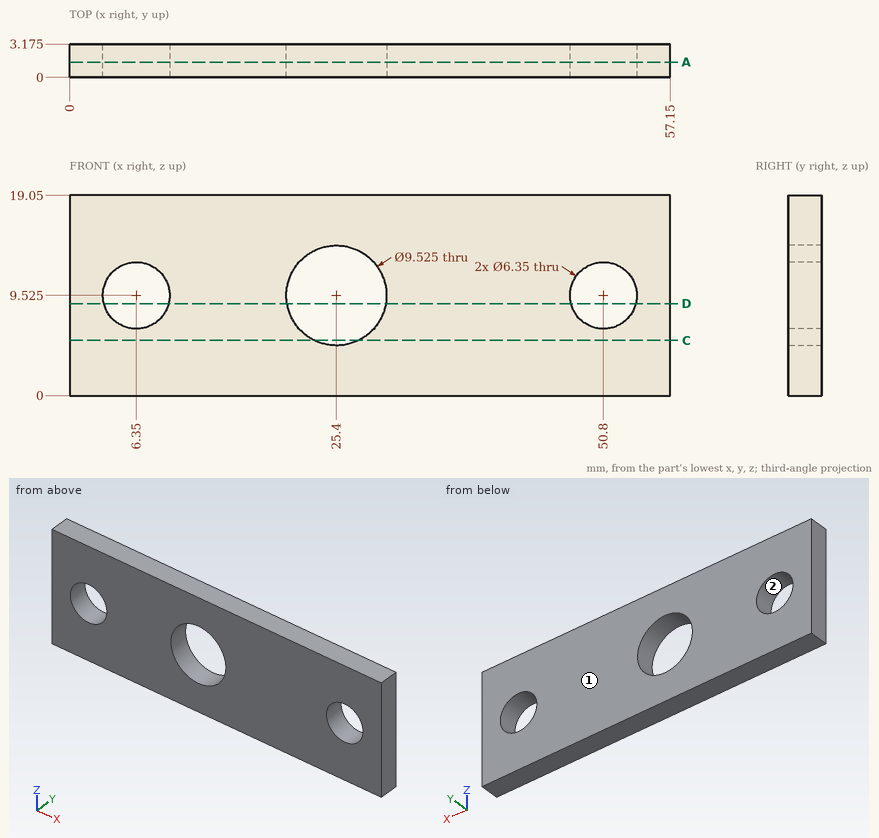
Answer from the drawing. Dimensions are ordinates in mm from the lowest x, y and z of the part. Give positions to 0.01 mm unless a question says otherwise; leave off trailing zeros. Loops run counter-clockwise (first coordinate to the right, second up) from the corner with the lowest first, then second, coordinate; pieces in that order, holes last.
Item 1: The part is cut by section A-A (y = 1.45). Give the number of separate pieces and of enclosed holes in the cut face, and give its area (3 significant figures).
Item 2: The part is cut by section C-C (z = 5.25). Write down the section's boundary in (x, y) (3 decimals).
Item 3: The part is cut by section D-D (z = 8.75). Write down the section's boundary in (x, y) (3 decimals).
Item 4: The mould has two halves that part along X. Classify the marked faces 1 and 2: released by +X, released by -X, zero draft, split by the parting line, or undercut.
Item 5: Find the intervals of material crossed by line 1 along X through (y, z) = (0.5, 9.5); line 2 along Z through (x, y) = (25.5, 0.1); line 3 along X through (y, z) = (1.8, 8.5) (3 decimals), in increasing order.
Taken from the geometry:
1. separate pieces: 1
1. enclosed holes: 3
1. area: 954 mm2
2. outline: (0, 0) - (23.301, 0) - (23.301, 3.175) - (0, 3.175) - close; (27.499, 0) - (57.15, 0) - (57.15, 3.175) - (27.499, 3.175) - close
3. outline: (0, 0) - (3.271, 0) - (3.271, 3.175) - (0, 3.175) - close; (9.429, 0) - (20.701, 0) - (20.701, 3.175) - (9.429, 3.175) - close; (30.099, 0) - (47.721, 0) - (47.721, 3.175) - (30.099, 3.175) - close; (53.879, 0) - (57.15, 0) - (57.15, 3.175) - (53.879, 3.175) - close
4. face 1: zero draft
4. face 2: undercut
5. line 1: x = 0 to 3.18, 9.52 to 20.64, 30.16 to 47.63, 53.97 to 57.15
5. line 2: z = 0 to 4.76, 14.29 to 19.05
5. line 3: x = 0 to 3.345, 9.355 to 20.749, 30.051 to 47.795, 53.805 to 57.15
